The listing builds one solid part. Answer for the finished solid, in the listing's coordinates (mm). A direction names the side the tool comes from. Coordinates: 2 decimals unless noted, no trailing zeros. Loops run counter-clockwise (first coordinate to the right, second up) from the corner with the lowest first, then second, coordinate; pieces in that order, holes last. Notation, with made-up numbers: (-38.75, -18.75) -> (3.25, -18.75) arc R34 ccw to (3.25, 14.25) -> close; hole circle Ø5 at (19.25, 65.25). An arc over 180 degrees is marked (long way). Answer in a Markdown table with one row per item.
```python
from build123d import *

# Parameters (mm, degrees)
BOSS_EXTRU_1_DEPTH = 5


with BuildPart() as part:
    # Esquisse1 → Boss.-Extru.1 (new body)
    with BuildSketch(Plane.XY):
        Polygon((-70, 40), (-72, 40), (-72, 30), (-84, 30), (-84, 25), (-82, 25), (-82, 26.5), (-77, 26.5), (-77, 25), (-72, 25), (-72, 15), (-77, 15), (-77, 13.5), (-82, 13.5), (-82, 15), (-84, 15), (-84, 10), (-72, 10), (-72, 0), (-70, 0), (-70, -5), (-65, -5), (-65, 0), (-55, 0), (-55, -5), (-50, -5), (-50, 0), (-30, 0), (-30, -5), (-25, -5), (-25, 0), (-15, 0), (-15, -5), (-10, -5), (-10, 0), (10, 0), (10, -5), (15, -5), (15, 0), (25, 0), (25, -5), (30, -5), (30, 0), (50, 0), (50, -5), (55, -5), (55, 0), (65, 0), (65, -5), (70, -5), (70, 0), (72, 0), (72, 10), (84, 10), (84, 15), (82, 15), (82, 13.5), (77, 13.5), (77, 15), (72, 15), (72, 25), (77, 25), (77, 26.5), (82, 26.5), (82, 25), (84, 25), (84, 30), (72, 30), (72, 40), (70, 40), (70, 45), (65, 45), (65, 40), (55, 40), (55, 45), (50, 45), (50, 40), (30, 40), (30, 45), (25, 45), (25, 40), (15, 40), (15, 45), (10, 45), (10, 40), (-10, 40), (-10, 45), (-15, 45), (-15, 40), (-25, 40), (-25, 45), (-30, 45), (-30, 40), (-50, 40), (-50, 45), (-55, 45), (-55, 40), (-65, 40), (-65, 45), (-70, 45), align=None)
    extrude(amount=BOSS_EXTRU_1_DEPTH)


solid = part.part
```
Item 1: A cutting plane is placed at A-A, the plane y = 38.5. Determine the outline of the cut face in (x, z), plus the area to 3 significant figures.
Findings below:
| item | result |
|---|---|
| outline | (-72, 0) -> (72, 0) -> (72, 5) -> (-72, 5) -> close |
| area | 720 mm2 |
Item 2: A tool of negligible diameter and unlimited length cuts with its end or side. For faces 5 (the face through (75, 15, 2)), 6 (the face through (30, -3, 2)), 7 (the face through (78, 30, 2)), from which of +Z, -Z, +X, -X, +Y, -Y can it reach the whole face along a straight path? Write none if from no direction.
Findings below:
| item | result |
|---|---|
| face 5 | +Z, -Z, +X |
| face 6 | +Z, -Z, -Y |
| face 7 | +Z, -Z, +X, +Y |
Item 3: Find the intervals of material crossed by probe 1 along X at (y, z) = (14.5, 1.05); probe 2 along Y at (x, z) = (77.5, 2.5); probe 3 along Y at (x, z) = (21, 1.25), in increasing order.
Findings below:
| item | result |
|---|---|
| probe 1 | x = -84 to -82, -77 to 77, 82 to 84 |
| probe 2 | y = 10 to 13.5, 26.5 to 30 |
| probe 3 | y = 0 to 40 |
Item 4: Flat-ended cylindrical pins translate along their axes: pin 1 Ø2.5 at (x, z) = (79, 1.5) entering from +Y; pin 2 Ø1.5 at (y, z) = (43, 1.5) entering from +X; pin 3 Ø2.5 at (y, z) = (43.5, 1.5) entering from -X. Find the tip coordinate at first contact, or state that the pin passes through.
Findings below:
| item | result |
|---|---|
| pin 1 | stops at y = 30 |
| pin 2 | stops at x = 70 |
| pin 3 | stops at x = -70 |
Item 5: Determine the mould class of faces 1 (the face through (-78, 30, 2)), 2 (the face through (-70, 43, 2)), 3 (the face through (20, 40, 2)), 4 (the face through (72, 5, 2)) for opening direction X: +X half, -X half, draft (parallel to the pull), parting line (faces both ways), or undercut.
Findings below:
| item | result |
|---|---|
| face 1 | draft |
| face 2 | -X half |
| face 3 | undercut |
| face 4 | +X half |
Item 6: A cutting plane is placed at B-B, the plane x = 40. Determine the outline of the cut face in (y, z).
Findings below:
| item | result |
|---|---|
| outline | (0, 0) -> (40, 0) -> (40, 5) -> (0, 5) -> close |
